Here's how the part is built. I have some questions about the finished solid (model axes, mm). Face numbers are marked on the shaded views. Give positions to 0.01 mm unless a question says otherwise; leave off trailing zeros. Loops run counter-clockwise (first coordinate to the right, second up) from the corner with the lowest first, then second, coordinate; pieces in that order, holes last. Notation, with made-up numbers: (-19, -10) -> (37, -10) arc R7 ccw to (37, -3) -> close; hole circle Ø5 at (13.5, -1). An arc over 180 degrees is marked (long way). Answer in a Markdown table with one row per item. Add a question column.
Item 1: If we section it at B-B (z = 10.25): Write out the boundary of the cut face in (x, y).
Item 2: If we section it at A-A (z = 16): Write out the boundary of the cut face in (x, y).
Item 3: We'd pull the mould along Y, two halves only. Please class the marked faces 1, 2 and 3: released by +Y, released by -Y, zero draft, split by the parting line, or undercut.
Item 4: For P1, Ø4, axis at x = -3.5, y = -6, coming from the -Z side; P2, Ø1.5, axis at x = -1, y = 0.5, coming from the -Z side; P3, Ø10, axis at x = 5, z = 13, coming from the -Y side; P4, Ø12, axis at y = -5.5, z = 9, coming from the +X side, each with a flat end and sliding along its axis, tell me the tip position at first contact or that it passes through.
Item 5: If I drill on line 1 (Y direction, x = -0.5, z = 24); line 2 (Y direction, x = -1, z = 11); line 3 (X direction, y = 7.5, z = 1.75), over which ranges is the centre line in solid material (lowest first)?
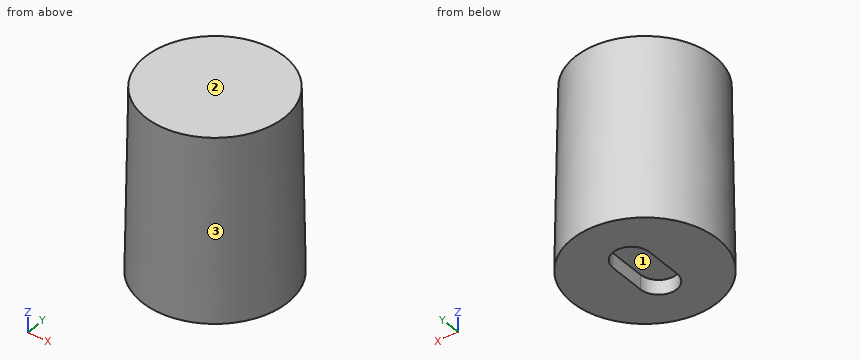
```python
from build123d import *

# Parameters (mm, degrees)
BASE_R         = 10
CYLINDER_DEPTH = 25
CYLINDER_TAPER = 1
KEY_SLOT_DEPTH = 2


# Read off the part's stored shape, not the designer's step: key slot
with BuildPart() as part:
    # base → cylinder (new body)
    with BuildSketch(Plane.XY):
        Circle(BASE_R)
    extrude(amount=CYLINDER_DEPTH, taper=CYLINDER_TAPER)

    # key slot outline → key slot (cut)
    with BuildSketch(Plane.XY):
        with BuildLine():
            Line((-2.5, 2.5), (-2.5, -2.5))
            ThreePointArc((-2.5, -2.5), (0, -5), (2.5, -2.5))
            Line((2.5, -2.5), (2.5, 2.5))
            ThreePointArc((2.5, 2.5), (0, 5), (-2.5, 2.5))
        make_face()
    extrude(amount=KEY_SLOT_DEPTH, mode=Mode.SUBTRACT)


solid = part.part
```
Recorded:
| question | item | result |
|---|---|---|
| 1 | outline | circle Ø19.64 at (0, 0) |
| 2 | outline | circle Ø19.44 at (0, 0) |
| 3 | face 1 | undercut |
| 3 | face 2 | zero draft |
| 3 | face 3 | split by the parting line |
| 4 | P1 | stops at z = 0 |
| 4 | P2 | stops at z = 2 |
| 4 | P3 | stops at y = -9.8 |
| 4 | P4 | stops at x = 9.89 |
| 5 | line 1 | y = -9.57 to 9.57 |
| 5 | line 2 | y = -9.76 to 9.76 |
| 5 | line 3 | x = -6.57 to 6.57 |
